```python
from build123d import *

# Parameters (mm, degrees)
SALIENTE_EXTRUIR1_DEPTH = 70
REDONDEO1_R             = 2
REDONDEO2_R             = 4


with BuildPart() as part:
    # Croquis1 → Saliente-Extruir1 (new body)
    with BuildSketch(Plane(origin=(0, 0, 0), x_dir=(0, 1, 0), z_dir=(0, 0, 1))):
        Polygon((-129.584937216, 88.672304845), (-90.389958144, 156.56), (90.389958144, 156.56), (129.584937216, 88.672304845), (132.183013428, 90.172304845), (92.122008952, 159.56), (-92.122008952, 159.56), (-132.183013428, 90.172304845), align=None)
    extrude(amount=SALIENTE_EXTRUIR1_DEPTH)

    # Redondeo1
    redondeo1_edges = [part.edges().sort_by_distance(p)[0] for p in [
        (-156.56, 90.389958144, 35),
        (-156.56, -90.389958144, 35),
    ]]
    fillet(redondeo1_edges, radius=REDONDEO1_R)

    # Redondeo2
    redondeo2_edges = [part.edges().sort_by_distance(p)[0] for p in [
        (-159.56, -92.122008952, 35),
        (-159.56, 92.122008952, 35),
    ]]
    fillet(redondeo2_edges, radius=REDONDEO2_R)


solid = part.part
```
Geometry: final body of the model. Coordinates: model frame, mm. A direction names the side the tool comes from. Round coordinates to 2 decimals unless told otherwise and drop trailing zeros. Order: outer loops, then holes, each group sorted by start corner. A loop starts at its lowest first (then second) coordinate and runs counter-clockwise, first axis right, second up. Notation, with made-up numbers: (-17, 28.25) -> (39, 28.25) arc R20 ccw to (39, 42.25) -> close; hole circle Ø1 at (5, 5). An arc over 180 degrees is marked (long way). Use CSV: the item, a comma, the result in double quotes. Start each with the question number.
1) Draft query along Y for faces 3 (the face through (-124.338, -112.458, 34.51)), 4 (the face through (-158, -1, 0)), 5 (the face through (-156.56, -1, 35)), 6 (the face through (-123.4, 113, 34.5)). Return one class per face: +Y half, -Y half, draft (parallel to the pull), parting line (faces both ways), or undercut.
2) Section B-B (z = 22.5). Return the cut outline in (x, y).
3) Material intervals for line 1 along X through (y, z) = (-30.5, 30.5); line 2 along Y through (x, z) = (-108, 36); line 3 along Y through (x, z) = (-93, 44), sorted ascending. Write a range as from..to.
4) Section D-D (y = 110.5). Return the cut outline in (x, z), and give its area (3 significant figures).
5) Section A-A (x = -139). Return the cut outline in (y, z).
6) Section C-C (y = -82.5). Return the cut outline in (x, z).
7) Set-up query: faces 1 (the face through (-122.58, 110.01, 34.51)), 2 (the face through (-158, -1, 70)). Return all of +Z, -Z, +X, -X, +Y, -Y with unobstructed straight access to the full face (end or side cutting, diameter ignored); none if empty.
8) First-contact query: pin 1 Ø4 at (y, z) = (-86, 43) entering from +X; pin 2 Ø6 at (x, z) = (-112, 16.5) entering from -Y; pin 3 Ø4 at (x, z) = (-151, 48) entering from -Y. Flat tips, straight axial feed; report the tip coordinate or a pass-through.
Returned:
1,face 3,"-Y half"
1,face 4,"draft"
1,face 5,"undercut"
1,face 6,"+Y half"
2,outline,"(-159.56, -89.81) arc R4 ccw to (-157.56, -93.28) -> (-90.17, -132.18) -> (-88.67, -129.58) -> (-155.56, -90.97) arc R2 cw to (-156.56, -89.24) -> (-156.56, 89.24) arc R2 cw to (-155.56, 90.97) -> (-88.67, 129.58) -> (-90.17, 132.18) -> (-157.56, 93.28) arc R4 ccw to (-159.56, 89.81) -> close"
3,line 1,"x = -159.56..-156.56"
3,line 2,"y = -121.89..-118.43, 118.43..121.89"
3,line 3,"y = -130.55..-127.09, 127.09..130.55"
4,outline,"(-127.73, 0) -> (-121.73, 0) -> (-121.73, 70) -> (-127.73, 70) -> close"
4,area,"420 mm²"
5,outline,"(-103.99, 0) -> (-100.53, 0) -> (-100.53, 70) -> (-103.99, 70) -> close; (100.53, 0) -> (103.99, 0) -> (103.99, 70) -> (100.53, 70) -> close"
6,outline,"(-159.56, 0) -> (-156.56, 0) -> (-156.56, 70) -> (-159.56, 70) -> close"
7,face 1,"+Z, -Z, +X"
7,face 2,"+Z, +X, -X, +Y, -Y"
8,pin 1,"stops at x = -156.56"
8,pin 2,"stops at y = -121.31"
8,pin 3,"stops at y = -98.22"
